The figure shows three views and two pictorial views of one solid part (mm, origin at its lowest corner). Answer the questions. Round coordinates to 2 decimals unless told otherwise and drop trailing zeros. Order: outer loops, then holes, each group sorted by start corner. A loop starts at its lowest first (then second) coordinate and runs counter-clockwise, first axis right, second up. Notation, with made-up numbers: (1, 45) - (16, 45) arc R19 cw to (16, 78) - close; hole circle Ø5 at (-31, 46). An arc over 180 degrees is marked (long way). Answer as a JSON object with one key per item and string values. Group by question number.
Q1. A cutting plane is placed at B-B on x = 19. Determine the outline of the cut face in (y, z), and give its area (3 significant figures).
Q2. Given pin 1 Ø1.2 at (y, z) = (1, 133.5) entering from -X; pin 2 Ø1.2 at (x, y) = (120, 2) entering from +Z; pin 3 Ø2 at (y, z) = (1.5, 35.5) entering from -X, each flat-ended and moving along its own axis, determine where each tip first touches the part or whether it passes through.
Q3. Consider line 1 (Z direction, x = 181, y = 2.25); line 2 (X direction, y = 2.45, z = 20); line 3 (X direction, y = 2.6, z = 116). Determine where each line is inside the solid, lowest interval first.
Q4. A cutting plane is placed at C-C on z = 20. Determine the outline of the cut face in (x, y), and give its area (3 significant figures).
Q5. A cutting plane is placed at D-D on y = 1.6. Count the separate pieces of the cut face and the enclosed holes in it, and give its area (3 significant figures).
Q6. A cutting plane is placed at A-A on x = 106.5. Determine the outline of the cut face in (y, z), and give its area (3 significant figures).
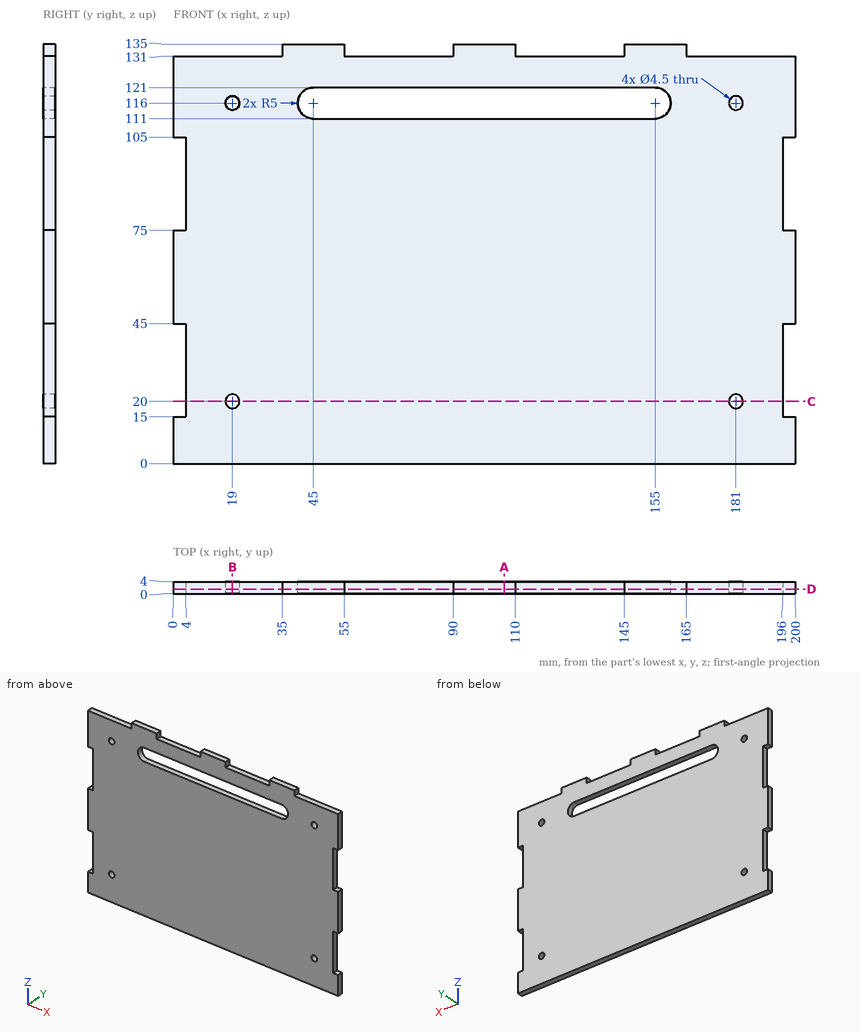
Result set:
{
 "1": {"outline": "(0, 0) - (4, 0) - (4, 17.75) - (0, 17.75) - close; (0, 22.25) - (4, 22.25) - (4, 113.75) - (0, 113.75) - close; (0, 118.25) - (4, 118.25) - (4, 131) - (0, 131) - close", "area": "488 mm²"},
 "2": {"pin 1": "stops at x = 35", "pin 2": "stops at z = 131", "pin 3": "stops at x = 4"},
 "3": {"line 1": "z = 0 to 17.75, 22.25 to 113.75, 118.25 to 131", "line 2": "x = 4 to 16.75, 21.25 to 178.75, 183.25 to 196", "line 3": "x = 0 to 16.75, 21.25 to 40, 160 to 178.75, 183.25 to 200"},
 "4": {"outline": "(4, 0) - (16.75, 0) - (16.75, 4) - (4, 4) - close; (21.25, 0) - (178.75, 0) - (178.75, 4) - (21.25, 4) - close; (183.25, 0) - (196, 0) - (196, 4) - (183.25, 4) - close", "area": "732 mm²"},
 "5": {"separate pieces": "1", "enclosed holes": "5", "area": "24,700 mm²"},
 "6": {"outline": "(0, 0) - (4, 0) - (4, 111) - (0, 111) - close; (0, 121) - (4, 121) - (4, 135) - (0, 135) - close", "area": "500 mm²"}
}
